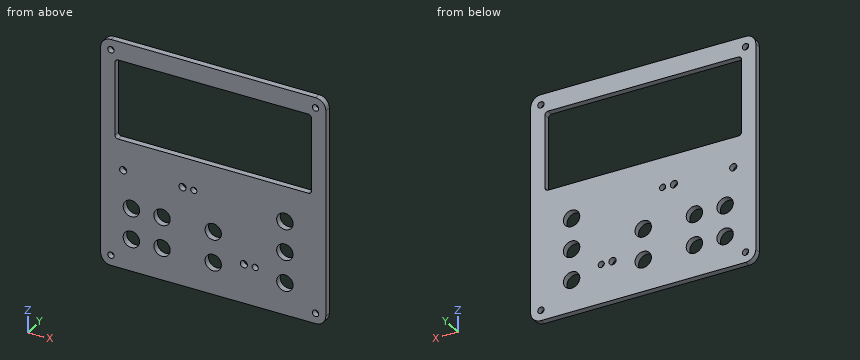
from build123d import *

# Parameters (mm, degrees)
SKETCH1_W           = 110
SKETCH1_H           = 110
SKETCH1_R           = 1.55
BOSS_EXTRUDE1_DEPTH = 3
FILLET1_R           = 5
SKETCH2_W           = 96
SKETCH2_H           = 38.5
CUT_EXTRUDE1_DEPTH  = 4
FILLET2_R           = 1.5
SKETCH3_R           = 4
CUT_EXTRUDE2_DEPTH  = 4
SKETCH4_R           = 1.75
SKETCH4_R_2         = 1.5
CUT_EXTRUDE3_DEPTH  = 4


with BuildPart() as part:
    # Sketch1 → Boss-Extrude1 (new body)
    with BuildSketch(Plane(origin=(0, 0, 0), x_dir=(1, 0, 0), z_dir=(0, 1, 0))):
        Rectangle(SKETCH1_W, SKETCH1_H)
        with Locations((-50, 50)):
            Circle(SKETCH1_R, mode=Mode.SUBTRACT)
        with Locations((50, 50)):
            Circle(SKETCH1_R, mode=Mode.SUBTRACT)
        with Locations((50, -50)):
            Circle(SKETCH1_R, mode=Mode.SUBTRACT)
        with Locations((-50, -50)):
            Circle(SKETCH1_R, mode=Mode.SUBTRACT)
    extrude(amount=BOSS_EXTRUDE1_DEPTH)

    # Fillet1
    fillet1_edges = [part.edges().sort_by_distance(p)[0] for p in [
        (-55, 1.5, -55),
        (55, 1.5, -55),
        (55, 1.5, 55),
        (-55, 1.5, 55),
    ]]
    fillet(fillet1_edges, radius=FILLET1_R)

    # Sketch2 → Cut-Extrude1 (cut, through all)
    with BuildSketch(Plane(origin=(0, 3, 0), x_dir=(1, 0, 0), z_dir=(0, 1, 0))):
        with Locations((0, -26.75)):
            Rectangle(SKETCH2_W, SKETCH2_H)
    extrude(amount=-CUT_EXTRUDE1_DEPTH, mode=Mode.SUBTRACT)

    # Fillet2
    fillet2_edges = [part.edges().sort_by_distance(p)[0] for p in [
        (-48, 1.5, 46),
        (-48, 1.5, 7.5),
        (48, 1.5, 7.5),
        (48, 1.5, 46),
    ]]
    fillet(fillet2_edges, radius=FILLET2_R)

    # Sketch3 → Cut-Extrude2 (cut, through all)
    with BuildSketch(Plane(origin=(0, 3, 0), x_dir=(1, 0, 0), z_dir=(0, 1, 0))):
        with Locations((-40, 39.5)):
            Circle(SKETCH3_R)
        with Locations((-40, 24.5)):
            Circle(SKETCH3_R)
        with Locations((-25, 39.5)):
            Circle(SKETCH3_R)
        with Locations((-25, 24.5)):
            Circle(SKETCH3_R)
        with Locations((0, 39.5)):
            Circle(SKETCH3_R)
        with Locations((0, 24.5)):
            Circle(SKETCH3_R)
        with Locations((35, 39.5)):
            Circle(SKETCH3_R)
        with Locations((35, 24.5)):
            Circle(SKETCH3_R)
        with Locations((35, 9.5)):
            Circle(SKETCH3_R)
    extrude(amount=-CUT_EXTRUDE2_DEPTH, mode=Mode.SUBTRACT)

    # Sketch4 → Cut-Extrude3 (cut, through all)
    with BuildSketch(Plane(origin=(0, 3, 0), x_dir=(1, 0, 0), z_dir=(0, 1, 0))):
        with Locations((-44, 7)):
            Circle(SKETCH4_R)
        with Locations((-15, 7)):
            Circle(SKETCH4_R)
        with Locations((-9.5, 7)):
            Circle(SKETCH4_R_2)
        with Locations((15, 36)):
            Circle(SKETCH4_R)
        with Locations((20.5, 36)):
            Circle(SKETCH4_R_2)
    extrude(amount=-CUT_EXTRUDE3_DEPTH, mode=Mode.SUBTRACT)


solid = part.part
Read the model definition and answer for the solid it produces. Units are mm, in the model's axes. Give positions to 0.01 mm unless a question says otherwise; leave off trailing zeros. Write each loop counter-clockwise with the first axis right and the second up, starting at its lowest first coordinate (ties: lowest second). Pieces come first, ordered by that corner, then holes. Notation, with made-up numbers: (-15, -20) - (3, -20) arc R11 cw to (3, -5) - close; hole circle Ø7 at (-10.75, -1). An arc over 180 degrees is marked (long way). Return JSON: item names as keys, results as strings.
Q1. A cutting plane is placed at C-C, the plane x = -32.5. Determine the outline of the cut face in (y, z).
Reply:
{"outline": "(0, -55) - (3, -55) - (3, 7.5) - (0, 7.5) - close; (0, 46) - (3, 46) - (3, 55) - (0, 55) - close"}
Q2. A cutting plane is placed at B-B, the plane z = -39.5. Determine the outline of the cut face in (x, y), and give its area (3 significant figures).
Reply:
{"outline": "(-55, 0) - (-44, 0) - (-44, 3) - (-55, 3) - close; (-36, 0) - (-29, 0) - (-29, 3) - (-36, 3) - close; (-21, 0) - (-4, 0) - (-4, 3) - (-21, 3) - close; (4, 0) - (31, 0) - (31, 3) - (4, 3) - close; (39, 0) - (55, 0) - (55, 3) - (39, 3) - close", "area": "234 mm²"}
Q3. Consider line 1 along Z through (x, y) = (35, 2); line 2 along X through (y, z) = (2.3, -39.5); line 3 along Z through (x, y) = (0, 2.1). Determine where each line is inside the solid, lowest interval first. Write a range as [from, to].
Reply:
{"line 1": "[-55, -43.5], [-35.5, -28.5], [-20.5, -13.5], [-5.5, 7.5], [46, 55]", "line 2": "[-55, -44], [-36, -29], [-21, -4], [4, 31], [39, 55]", "line 3": "[-55, -43.5], [-35.5, -28.5], [-20.5, 7.5], [46, 55]"}
Q4. A cutting plane is placed at A-A, the plane x = -15. Determine the outline of the cut face in (y, z).
Reply:
{"outline": "(0, -55) - (3, -55) - (3, -8.75) - (0, -8.75) - close; (0, -5.25) - (3, -5.25) - (3, 7.5) - (0, 7.5) - close; (0, 46) - (3, 46) - (3, 55) - (0, 55) - close"}
Q5. A cutting plane is placed at D-D, the plane z = 32. Determine the outline of the cut face in (x, y), and give its area (3 significant figures).
Reply:
{"outline": "(-55, 0) - (-48, 0) - (-48, 3) - (-55, 3) - close; (48, 0) - (55, 0) - (55, 3) - (48, 3) - close", "area": "42.0 mm²"}
Q6. Given P1, Ø2.5, axis at x = -9.5, z = -7, coming from the +Y side, flat-ended and moving along its own axis, determine where the tip first touches the part or whether it passes through.
Reply:
{"P1": "through"}
